The figure shows three views and two pictorial views of one solid part (mm, origin at its lowest corner). Answer the questions. A direction names the side the tool comes from. Give positions to 0.01 mm unless a question says otherwise; leave off trailing zeros. Order: outer loops, then holes, each group sorted by start corner. A loop starts at its lowest first (then second) coordinate and runs counter-clockwise, first axis right, second up. Notation, with made-up numbers: (60.25, 37.25) - (82.25, 37.25) arc R8 ccw to (82.25, 41.25) - close; hole circle Ø6 at (45, 37.25). An arc over 180 degrees is marked (long way). Write item = value, one per line.
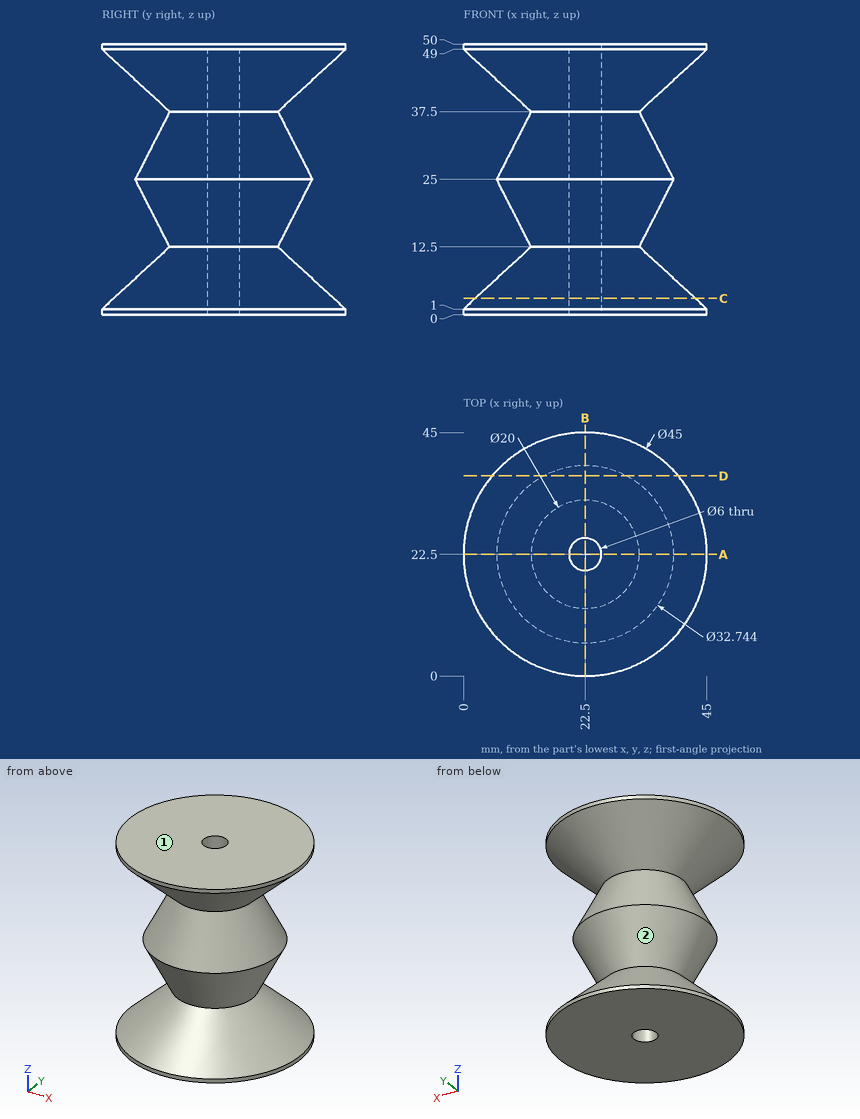
1. For the marked faces 1 and 2, determine the directions among +Z, -Z, +X, -X, +Y, -Y from which every point of the face is accessible in a straight line to the end or side of a thin tool.
Recorded:
face_1 = +Z, +X, -X, +Y, -Y
face_2 = none
2. Flat-ended cylindrical pins translate along their axes: pin 1 (3 mm diameter, centred on y = 25.5, z = 41, fed in from -X) (1 decimal); pin 2 (2 mm diameter, centred on y = 9.5, z = 29, fed in from -X); pin 3 (8 mm diameter, centred on x = 16.5, z = 43.5, fed in from +Y); pin 4 (2 mm diameter, centred on x = 16.5, y = 20.5, fed in from -Z). Find the tip coordinate at first contact, or state that the pin passes through.
Recorded:
pin_1 = 7.3
pin_2 = 14.4
pin_3 = 42.62
pin_4 = 0
3. Straight lines are drawn through the part: L1, parallel to Z at x = 22.5, y = 7.5; L2, parallel to Z at x = 14.5, y = 13.5 (1 decimal); L3, parallel to X at y = 22, z = 25 (1 decimal). For each, find the intervals that lie inside material, in ascending order. Write a range as [from, to].
Recorded:
L1 = [0, 7.9], [22.31, 27.69], [42.1, 50]
L2 = [0, 10.6], [16.5, 33.5], [39.4, 50]
L3 = [6.1, 19.5], [25.5, 38.9]
4. Section A-A (y = 22.5) is taken. Determine the outline of the cut face in (x, z), and give its area (3 significant figures).
Recorded:
outline = (0, 0) - (19.5, 0) - (19.5, 50) - (0, 50) - (0, 49) - (12.5, 37.5) - (6.13, 25) - (12.5, 12.5) - (0, 1) - close; (25.5, 0) - (45, 0) - (45, 1) - (32.5, 12.5) - (38.87, 25) - (32.5, 37.5) - (45, 49) - (45, 50) - (25.5, 50) - close
area = 1,200 mm^2
5. Section C-C (z = 3) is taken. Determine the outline of the cut face in (x, y), and give its area (3 significant figures).
Recorded:
outline = circle Ø40.65 at (22.5, 22.5); hole circle Ø6 at (22.5, 22.5)
area = 1,270 mm^2
6. Section D-D (y = 37) is taken. Count the separate pieces of the cut face and the enclosed holes in it, and give its area (3 significant figures).
Recorded:
separate_pieces = 3
enclosed_holes = 0
area = 465 mm^2
